The model under review builds one solid part; all positions refer to its coordinate system, in mm. A direction names the side the tool comes from. Give positions to 0.01 mm unless a question says otherwise; leave off trailing zeros. Order: outer loops, then holes, each group sorted by start corner. A loop starts at its lowest first (then second) coordinate and runs counter-clockwise, first axis right, second up. Notation, with made-up numbers: (45.5, 11.25) - (80.5, 11.25) arc R10 ccw to (80.5, 27.25) - close; hole circle Ø7 at (25.5, 82). An arc over 180 degrees is marked (long way). Write item = value, one per line. Start each with the question number.
1. Machinability: for faces 5 (the cylindrical face through (16.133, -60.711, 4.785)), 6 (the flat face through (3.175, -61, 20)), 7 (the flat face through (6.35, -38, 34)), which of the approach directions +Z, -Z, +X, -X, +Y, -Y give a long, thin tool a straight path to every point of the face, cutting with its end or side? Answer none if there is none.
2. We need section C-C, the plane y = -38.1. Give the boundary of the cut face in (x, z) (3 decimals).
3. For P1, Ø2.5, axis at y = -11.5, z = 23.5, coming from the +X side; P2, Ø11.5, axis at y = -24, z = 22, coming from the +X side; P3, Ø9, axis at x = 17, y = -13.5, coming from the +Z side, all flat-tipped, find the tip position at first contact; note any pin that passes through.
4. We need section D-D, the plane x = 18. Give the boundary of the cut face in (y, z) (3 decimals), and give its area (3 significant figures).
5. We need section A-A, the plane z = 22.86. State how many separate pieces and enclosed holes the cut face has, and give its area (3 significant figures).
6. Mouldability with a two-part tool opening along X and no side actions: class faces 1 (the flat face through (31.75, -38, 3)), 2 (the flat face through (0, -29, 18)), 3 (the cylindrical face through (17.47, -60.82, 1.57)), 4 (the flat face through (19, -38, 6.35)) as pulls with the +X half, pulls with the -X half, needs draft (parallel to the pull), parting line crosses it, or undercut.
7. Wall thickness on probe 1 along Z at (x, y) = (4.15, -12.7); probe 2 along Y at (x, z) = (3.5, 20); probe 3 along Z at (x, y) = (30.5, -32): over which ranges is each line inside the solid? List them lowest first.
from build123d import *

# Parameters (mm, degrees)
F1_DEPTH             = 76.2
F5_D                 = 6.35
F5_CBORE_D           = 8.255
F5_CBORE_DEPTH       = 3.175
F5_ON_F4_D           = 6.35
F5_ON_F4_CBORE_D     = 8.255
F5_ON_F4_CBORE_DEPTH = 3.175
F6_D                 = 19.05


with BuildPart() as f1:
    # F0 (on Front) → F1 (new body)
    with BuildSketch(Plane.XZ):
        Polygon((0, 44.45), (0, 0), (31.75, 0), (31.75, 6.35), (6.35, 6.35), (6.35, 44.45), align=None)
    extrude(amount=F1_DEPTH)

    # F5 (through all)
    with Locations(Plane.YZ.offset(6.35)):
        with Locations((-63.5, 22.86), (-12.7, 22.86)):
            CounterBoreHole(F5_D / 2, F5_CBORE_D / 2, F5_CBORE_DEPTH)

    # F5 on F4 (through all)
    with Locations(Plane.XY.offset(6.35)):
        with Locations((19.1747965182, -12.7), (19.1747965182, -63.5006131711)):
            CounterBoreHole(F5_ON_F4_D / 2, F5_ON_F4_CBORE_D / 2, F5_ON_F4_CBORE_DEPTH)

    # F6 (through all)
    with Locations(Plane.YZ.offset(6.35)):
        with Locations((-38.1, 22.86)):
            Hole(F6_D / 2)


solid = f1.part
Model answer:
q1.face_5 = +Z
q1.face_6 = +X
q1.face_7 = +Z, +X, +Y, -Y
q2.outline = (0, 0) - (31.75, 0) - (31.75, 6.35) - (6.35, 6.35) - (6.35, 13.335) - (0, 13.335) - close; (0, 32.385) - (6.35, 32.385) - (6.35, 44.45) - (0, 44.45) - close
q3.P1 = through
q3.P2 = 6.35
q3.P3 = 6.35
q4.outline = (-76.2, 0) - (-66.45, 0) - (-66.45, 3.175) - (-67.457, 3.175) - (-67.457, 6.35) - (-76.2, 6.35) - close; (-60.551, 0) - (-15.65, 0) - (-15.65, 3.175) - (-16.657, 3.175) - (-16.657, 6.35) - (-59.544, 6.35) - (-59.544, 3.175) - (-60.551, 3.175) - close; (-9.75, 0) - (0, 0) - (0, 6.35) - (-8.743, 6.35) - (-8.743, 3.175) - (-9.75, 3.175) - close
q4.area = 396 mm2
q5.separate_pieces = 4
q5.enclosed_holes = 0
q5.area = 270 mm2
q6.face_1 = pulls with the +X half
q6.face_2 = pulls with the -X half
q6.face_3 = undercut
q6.face_4 = needs draft
q7.probe_1 = 0 to 18.73, 26.99 to 44.45
q7.probe_2 = -76.2 to -66.48, -60.52 to -47.19, -29.01 to -15.68, -9.72 to 0
q7.probe_3 = 0 to 6.35
